Autodesk Inventor part; units mm, degrees
ref_plane "YZ Plane" through (0, 0, 0) normal (1, 0, 0) x (0, 1, 0)
ref_plane "XZ Plane" through (0, 0, 0) normal (0, 1, 0) x (-1, 0, 0)
ref_plane "XY Plane" through (0, 0, 0) normal (0, 0, 1) x (1, 0, 0)
sketch "Sketch1" plane through (0, 0, 0) normal (0, 0, 1) x (1, 0, 0)
  line L0 (-26, -3.6985) -> (-3.6985, -26)
  line L1 (-3.6985, -26) -> (3.6985, -26)
  line L2 (3.6985, -26) -> (26, -3.6985)
  line L3 (26, -3.6985) -> (26, 3.6985)
  line L4 (26, 3.6985) -> (3.6985, 26)
  line L5 (3.6985, 26) -> (-3.6985, 26)
  line L6 (-3.6985, 26) -> (-26, 3.6985)
  line L7 (-26, 3.6985) -> (-26, -3.6985)
  circle A0 centre (0, 0) radius 5
  line L8 (-21, 0) -> (0, -21) construction
  line L9 (0, -21) -> (21, 0) construction
  line L10 (21, 0) -> (0, 21) construction
  line L11 (0, 21) -> (-21, 0) construction
  circle A1 centre (0, 21) radius 2.25
  circle A2 centre (-21, 0) radius 2.25
  circle A3 centre (0, -21) radius 2.25
  circle A4 centre (21, 0) radius 2.25
  point P0 (0, 26)
  point P1 (26, 0)
  dimension "d0" = 10
  dimension "d1" = 42
  dimension "d2" = 135
  dimension "d3" = 42
  dimension "d4" = 4.5
  dimension "d5" = 52
extrude "Extrusion1" add sketch "Sketch1" along normal blind 10
sketch "Sketch2" plane through (0, 0, 10) normal (0, 0, 1) x (1, 0, 0)
  circle A0 centre (0, 0) radius 5
  circle A1 centre (0, 0) radius 17
  dimension "d8" = 34
extrude "Extrusion2" add sketch "Sketch2" along normal blind 17
sketch "Sketch3" plane through (0, 0, 0) normal (0, 0, -1) x (-1, 0, 0)
  circle A0 centre (0, 21) radius 4
  circle A1 centre (21, 0) radius 4
  circle A2 centre (0, -21) radius 4
  circle A3 centre (-21, 0) radius 4
  circle A4 centre (0, 21) radius 2.25
  circle A5 centre (-21, 0) radius 2.25
  circle A6 centre (21, 0) radius 2.25
  circle A7 centre (0, -21) radius 2.25
  point P0 (0, 0)
  dimension "d11" = 8
extrude "Extrusion3" cut sketch "Sketch3" against normal blind 4 contours A0 | A1 | A2 | A3 | A4 | A5 | A6 | A7
sketch "Sketch5" plane through (0, 0, 27) normal (0, 0, 1) x (1, 0, 0)
  line L0 (-9.8137, 1.5) -> (-1.5, 9.8137)
  line L1 (-1.5, 9.8137) -> (1.5, 9.8137)
  line L2 (1.5, 9.8137) -> (9.8137, 1.5)
  line L3 (9.8137, 1.5) -> (9.8137, -1.5)
  line L4 (9.8137, -1.5) -> (1.5, -9.8137)
  line L5 (1.5, -9.8137) -> (-1.5, -9.8137)
  line L6 (-1.5, -9.8137) -> (-9.8137, -1.5)
  line L7 (-9.8137, -1.5) -> (-9.8137, 1.5)
  circle A0 centre (0, 0) radius 5
  point P0 (9.8137, 0)
  point P1 (-9.8137, 0)
  point P2 (0, 9.8137)
  point P3 (0, -9.8137)
  dimension "d14" = 16
  dimension "d15" = 3
  dimension "d16" = 10
extrude "Extrusion4" add sketch "Sketch5" along normal blind 8.5
properties part number "FK10"
Here's how the part is built. I have some questions about the finished solid (model axes, mm). A direction names the side the tool comes from. Give positions to 0.01 mm unless a question says otherwise; leave off trailing zeros. Order: outer loops, then holes, each group sorted by start corner. A loop starts at its lowest first (then second) coordinate and runs counter-clockwise, first axis right, second up. Notation, with made-up numbers: M -29,30.5 L -22,30.5 A20 ccw -22,42.5 Z; hole C -14.5,-6 d2. An arc over 180 degrees is marked long. Answer as a JSON object with one key per item and string values. Group by question number.
1) On a 3-axis mill with a long thin cutter (end or side, diameter ignored), from which of +Z, -Z, +X, -X, +Y, -Y can I reach the whole of each face in a straight line? I mean faces 1 (the flat face through (-9.814, 0, 31)), 2 (the flat face through (9.814, 0, 31)), 3 (the flat face through (4, 8, 27)), 4 (the cylindrical face through (24.2, -2.4, 2)), 5 (the flat face through (-5.715, 5.599, 31.19)). Say none if no direction works.
2) Please list where these lines run through material, in increasing order: L1, parallel to Y at x = -1.5, z = 9; L2, parallel to Z at x = -13, y = 3.5; L3, parallel to Z at x = 15, y = 13. Write a range as [from, to].
3) We'd pull the mould along Y, two halves only. Please class faces 6 (the cylindrical face through (23.146, -0.676, 6.958)), 7 (the flat face through (-26, 0, 5)), 8 (the flat face through (5.599, 5.715, 31.19)): pulls with the +Y half, pulls with the -Y half, needs draft (parallel to the pull), parting line crosses it, or undercut.
4) Suppose I cut it at D-D, the plane z = 3. Write out the boundary of the cut face in (x, y).
5) Suppose I cut it at B-B, the plane z = 28. Write out the boundary of the cut face in (x, y), plus the area to 3 significant figures.
6) I'm going to push flat-ended pins straight in: pin 1 Ø2.5 at (x, z) = (0, 33) entering from +Y; pin 2 Ø3 at (x, y) = (-10.5, -9.5) entering from +Z; pin 3 Ø4 at (x, y) = (21, 0) entering from +Z; pin 4 Ø7 at (x, y) = (21, 0) entering from +Z. Where does each tip first touch, or does it pass through?
7) Suppose I cut it at A-A, the plane x = 0. Count the separate pieces of the cut face and the enclosed holes in it, plus the area to 3 significant figures.
Results found:
{
 "1": {"face 1": "+Z, -X, +Y, -Y", "face 2": "+Z, +X, +Y, -Y", "face 3": "+Z", "face 4": "-Z", "face 5": "+Z, -X, +Y"},
 "2": {"L1": "[-26, -22.68], [-19.32, -4.77], [4.77, 19.32], [22.68, 26]", "L2": "[0, 27]", "L3": "[0, 10]"},
 "3": {"face 6": "undercut", "face 7": "needs draft", "face 8": "pulls with the +Y half"},
 "4": {"outline": "M -26,-3.7 L -3.7,-26 L 3.7,-26 L 26,-3.7 L 26,3.7 L 3.7,26 L -3.7,26 L -26,3.7 Z; hole C -21,0 d8; hole C 0,0 d10; hole C 0,-21 d8; hole C 0,21 d8; hole C 21,0 d8"},
 "5": {"outline": "M -9.81,-1.5 L -1.5,-9.81 L 1.5,-9.81 L 9.81,-1.5 L 9.81,1.5 L 1.5,9.81 L -1.5,9.81 L -9.81,1.5 Z; hole C 0,0 d10", "area": "168 mm²"},
 "6": {"pin 1": "y = 9.81", "pin 2": "z = 27", "pin 3": "through", "pin 4": "z = 10"},
 "7": {"separate pieces": "4", "enclosed holes": "0", "area": "792 mm²"}
}
